Source: CAD feature listing. Evaluate the final solid. Frame: model axes, mm. Round coordinates to 2 decimals unless told otherwise and drop trailing zeros. Loops run counter-clockwise (first coordinate to the right, second up) from the corner with the lowest first, then second, coordinate; pieces in that order, holes last. Notation, with made-up numbers: (-30, 6.5) -> (28, 6.5) arc R31 cw to (28, 43.5) -> close; hole circle Ø4 at (-1, 23.5). An arc over 180 degrees is marked (long way). Put each result on its own line as item: value. Start each with the question number.
1. Cut plane B-B (y = -9.9). Return the cut outline in (x, z), then the cut area to 3 significant figures.
2. Cut plane D-D (y = 8.25). Return the cut outline in (x, z), then the cut area to 3 significant figures.
3. Cut plane A-A (x = 29.8). Return the cut outline in (y, z), then the cut area to 3 significant figures.
4. Cut plane C-C (z = 4.5). Return the cut outline in (x, y).
5. Material intervals for L1, parallel to X at y = -11, z = 7.75; L2, parallel to Y at x = -29.8, z = 4.25; L3, parallel to Y at x = 28.5, z = 6, sorted ascending.
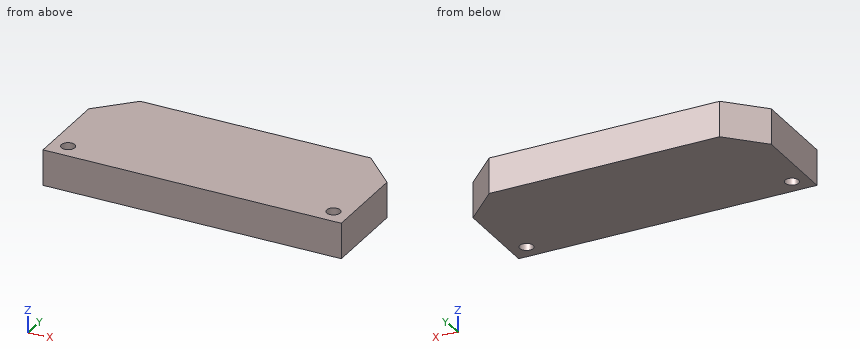
```python
from build123d import *

# Parameters (mm, degrees)
SKETCH1_W           = 67
SKETCH1_H           = 27.2
BOSS_EXTRUDE1_DEPTH = 8
SKETCH3_R           = 1.5
CUT_EXTRUDE1_DEPTH  = 8
CHAMFER1_SIZE       = 7.6


with BuildPart() as part:
    # Sketch1 → Boss-Extrude1 (new body)
    with BuildSketch(Plane.XY):
        Rectangle(SKETCH1_W, SKETCH1_H)
    extrude(amount=BOSS_EXTRUDE1_DEPTH)

    # Sketch3 → Cut-Extrude1 (cut)
    with BuildSketch(Plane.XY.offset(8)):
        with Locations((29.8, -9.9)):
            Circle(SKETCH3_R)
        with Locations((-29.8, -9.9)):
            Circle(SKETCH3_R)
    extrude(amount=-CUT_EXTRUDE1_DEPTH, mode=Mode.SUBTRACT)

    # Chamfer1
    chamfer1_edges = [part.edges().sort_by_distance(p)[0] for p in [
        (-33.5, 13.6, 4),
        (33.5, 13.6, 4),
    ]]
    chamfer(chamfer1_edges, length=CHAMFER1_SIZE)


solid = part.part
```
Solution:
1. outline: (-33.5, 0) -> (-31.3, 0) -> (-31.3, 8) -> (-33.5, 8) -> close; (-28.3, 0) -> (28.3, 0) -> (28.3, 8) -> (-28.3, 8) -> close; (31.3, 0) -> (33.5, 0) -> (33.5, 8) -> (31.3, 8) -> close
1. area: 488 mm^2
2. outline: (-31.25, 0) -> (31.25, 0) -> (31.25, 8) -> (-31.25, 8) -> close
2. area: 500 mm^2
3. outline: (-13.6, 0) -> (-11.4, 0) -> (-11.4, 8) -> (-13.6, 8) -> close; (-8.4, 0) -> (9.7, 0) -> (9.7, 8) -> (-8.4, 8) -> close
3. area: 162 mm^2
4. outline: (-33.5, -13.6) -> (33.5, -13.6) -> (33.5, 6) -> (25.9, 13.6) -> (-25.9, 13.6) -> (-33.5, 6) -> close; hole circle Ø3 at (-29.8, -9.9); hole circle Ø3 at (29.8, -9.9)
5. L1: x = -33.5 to -30.82, -28.78 to 28.78, 30.82 to 33.5
5. L2: y = -13.6 to -11.4, -8.4 to 9.7
5. L3: y = -13.6 to -10.65, -9.15 to 11
